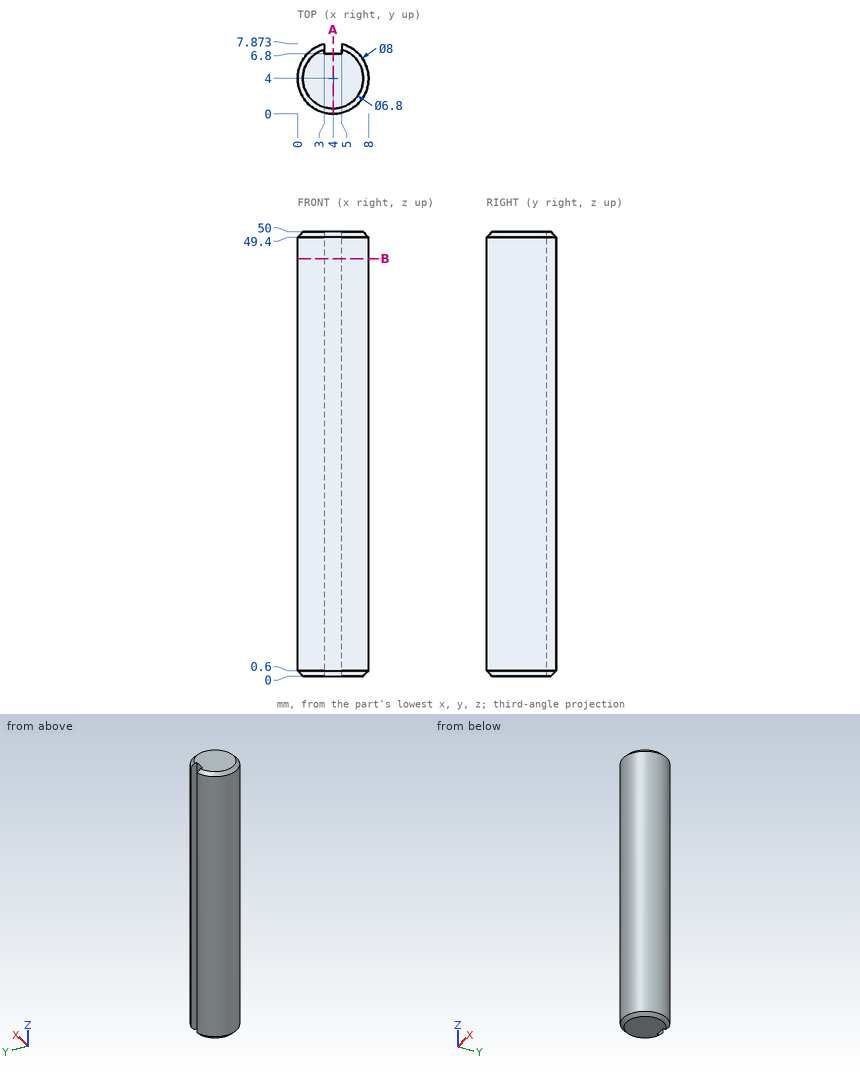
Could you check a few things on this drawing? It's one solid part, dimensions in mm from its lowest x, y, z. Give positions to 0.01 mm unless a question says otherwise; leave off trailing zeros. Write each loop counter-clockwise with the first axis right and the second up, starting at its lowest first coordinate (ties: lowest second). Pieces come first, ordered by that corner, then holes. Notation, with made-up numbers: (31, 2) - (67, 2) arc R29 ccw to (67, 25) - close; hole circle Ø1 at (-11.75, 70.25). An arc over 180 degrees is marked (long way). Use CSV: the item, a comma, the result in double quotes. Start each with the question number.
Item 1: I want a section at A-A, the plane x = 4. Please give me the cut outline in (y, z), then the cut area to 3 significant figures.
Item 2: If I drill on line 1 along X through (y, z) = (7, 31); line 2 along Z through (x, y) = (7.75, 3.75); line 3 along Y through (x, z) = (6.25, 11), over which ranges is the centre line in solid material (lowest first)?
Item 3: I want a section at B-B, the plane z = 47. Please give me the cut outline in (x, y).
Item 4: I'm going to push flat-ended pins straight in: pin 1 (4 mm diameter, centred on x = 7, z = 13.5, fed in from -Y); pin 2 (1.2 mm diameter, centred on y = 7, z = 16.5, fed in from -X); pin 3 (1.5 mm diameter, centred on x = 4, z = 7, fed in from +Y); pin 4 (3 mm diameter, centred on x = 2.5, z = 8, fed in from -Y). Where does each tip first touch, or does it pass through?
Findings:
1,outline,"(0, 0.6) - (0.6, 0) - (6.8, 0) - (6.8, 50) - (0.6, 50) - (0, 49.4) - close"
1,area,"340 mm2"
2,line 1,"x = 1.35 to 3, 5 to 6.65"
2,line 2,"z = 0.36 to 49.64"
2,line 3,"y = 0.69 to 7.31"
3,outline,"(3, 6.8) - (3, 7.87) arc R4 ccw (long way) to (5, 7.87) - (5, 6.8) - close"
4,pin 1,"stops at y = 0.13"
4,pin 2,"stops at x = 0.8"
4,pin 3,"stops at y = 6.8"
4,pin 4,"stops at y = 0"
